Design review of the part shown in the three views and the two pictorial views. Dimensions are in mm from the part's minimum x, y and z. Give positions to 0.01 mm unless a question says otherwise; leave off trailing zeros. Order: outer loops, then holes, each group sorted by start corner. A loop starts at its lowest first (then second) coordinate and runs counter-clockwise, first axis right, second up. Notation, with made-up numbers: (4.5, -33.75) -> (49.5, -33.75) arc R15 ccw to (49.5, -6.75) -> close; hole circle Ø5 at (-23, 84). An arc over 180 degrees is marked (long way). Use one line per item in the form item = value.
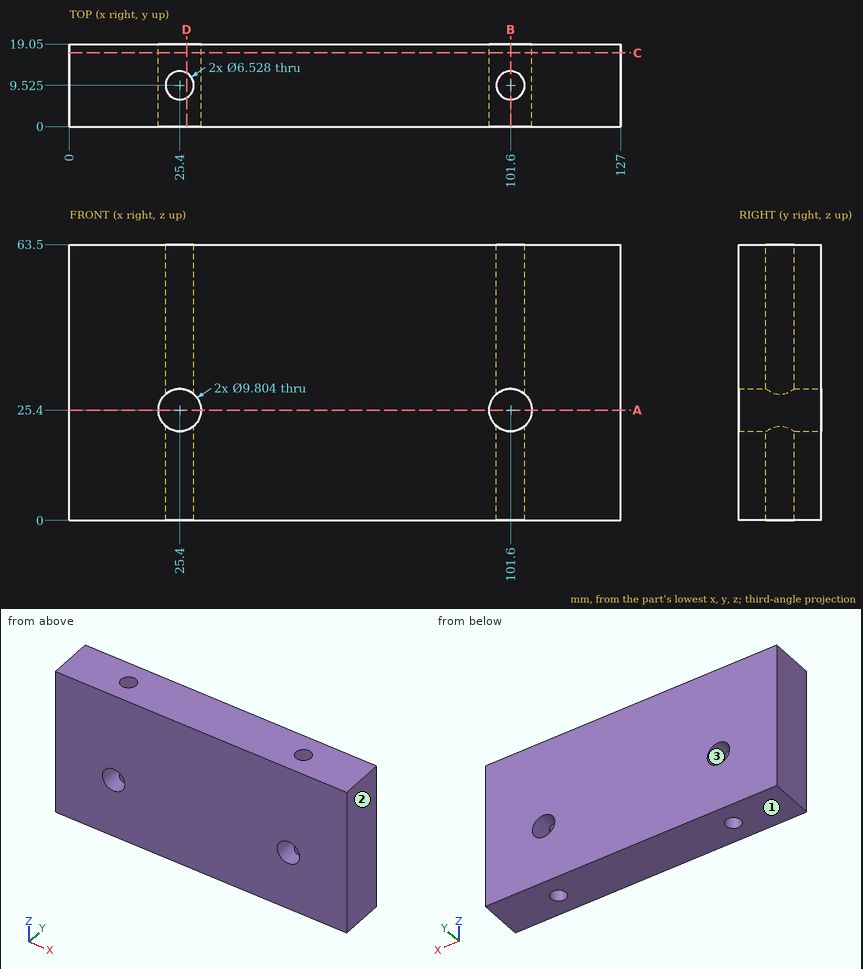
1. Add section A-A on z = 25.4. Give the boundary of the cut face in (x, y).
Values:
outline = (0, 0) -> (20.5, 0) -> (20.5, 19.05) -> (0, 19.05) -> close; (30.3, 0) -> (96.7, 0) -> (96.7, 19.05) -> (30.3, 19.05) -> close; (106.5, 0) -> (127, 0) -> (127, 19.05) -> (106.5, 19.05) -> close
2. The part is to be moulded in two halves that separate along Z. For the marked faces 1, 2 and 3, say which applies: +Z half, -Z half, draft (parallel to the pull), parting line (faces both ways), or undercut.
Values:
face_1 = -Z half
face_2 = draft
face_3 = undercut
3. Add section D-D on x = 27. Give the boundary of the cut face in (y, z).
Values:
outline = (0, 0) -> (6.68, 0) -> (6.68, 20.77) -> (0, 20.77) -> close; (0, 30.03) -> (6.68, 30.03) -> (6.68, 63.5) -> (0, 63.5) -> close; (12.37, 0) -> (19.05, 0) -> (19.05, 20.77) -> (12.37, 20.77) -> close; (12.37, 30.03) -> (19.05, 30.03) -> (19.05, 63.5) -> (12.37, 63.5) -> close
4. Add section C-C on y = 17. Give the boundary of the cut face in (x, z) (1 decimal).
Values:
outline = (0, 0) -> (127, 0) -> (127, 63.5) -> (0, 63.5) -> close; hole circle Ø9.8 at (25.4, 25.4); hole circle Ø9.8 at (101.6, 25.4)
5. For pin 1 Ø5 at (x, y) = (101.6, 9.525) entering from -Z; pin 2 Ø10.5 at (x, y) = (25.4, 9.525) entering from +Z, all flat-tipped, find the tip position at first contact; note any pin that passes through.
Values:
pin_1 = through
pin_2 = 63.5
6. For L1, parallel to X at y = 9.75, z = 48; L2, parallel to Y at x = 25.4, z = 5.5; L3, parallel to X at y = 5.75, z = 24, list the stretches that pass through material, from the lowest coordinate up.
Values:
L1 = 0 to 22.14, 28.66 to 98.34, 104.86 to 127
L2 = 0 to 6.26, 12.79 to 19.05
L3 = 0 to 20.7, 30.1 to 96.9, 106.3 to 127
7. Add section B-B on x = 101.6. Give the boundary of the cut face in (y, z).
Values:
outline = (0, 0) -> (6.26, 0) -> (6.26, 20.5) -> (0, 20.5) -> close; (0, 30.3) -> (6.26, 30.3) -> (6.26, 63.5) -> (0, 63.5) -> close; (12.79, 0) -> (19.05, 0) -> (19.05, 20.5) -> (12.79, 20.5) -> close; (12.79, 30.3) -> (19.05, 30.3) -> (19.05, 63.5) -> (12.79, 63.5) -> close
